from build123d import *

# Parameters (mm, degrees)
SKETCH1_R           = 1.397
SKETCH1_R_2         = 1.651
SKETCH1_R_3         = 1.016
SKETCH1_W           = 58.544107304
SKETCH1_H           = 8.89
SKETCH1_W_2         = 6.35
SKETCH1_H_2         = 3.175
BOSS_EXTRUDE1_DEPTH = 3.175


with BuildPart() as part:
    # Sketch1 → Boss-Extrude1 (new body)
    with BuildSketch(Plane(origin=(0, 0, 0), x_dir=(1, 0, 0), z_dir=(0, 1, 0))):
        with BuildLine():
            Line((38.407265908, 13.335), (41.582265908, 13.335))
            Line((41.582265908, 13.335), (50.342102347, 13.335))
            ThreePointArc((50.342102347, 13.335), (57.058059725, 24.74076345), (67.270928268, 33.160552015))
            ThreePointArc((67.270928268, 33.160552015), (-10.756431789, 74.224653419), (-73.916912814, 12.7))
            Line((-73.916912814, 12.7), (-73.916912814, -12.7))
            ThreePointArc((-73.916912814, -12.7), (-10.756431789, -74.224653419), (67.270928268, -33.160552015))
            ThreePointArc((67.270928268, -33.160552015), (60.584216496, -28.355013333), (55.086193863, -22.225))
            ThreePointArc((55.086193863, -22.225), (52.41895011, -17.937530518), (50.342102347, -13.335))
            Line((50.342102347, -13.335), (46.281265908, -13.335))
            Line((46.281265908, -13.335), (41.582265908, -13.335))
            Line((41.582265908, -13.335), (41.582265908, -22.86))
            Line((41.582265908, -22.86), (38.407265908, -22.86))
            Line((38.407265908, -22.86), (38.407265908, -13.335))
            Line((38.407265908, -13.335), (-2.486734092, -13.335))
            Line((-2.486734092, -13.335), (-2.486734092, -6.604))
            Line((-2.486734092, -6.604), (-38.046734092, -6.604))
            Line((-38.046734092, -6.604), (-38.046734092, 6.604))
            Line((-38.046734092, 6.604), (-2.486734092, 6.604))
            Line((-2.486734092, 6.604), (-2.486734092, 13.335))
            Line((-2.486734092, 13.335), (38.407265908, 13.335))
        make_face()
        with Locations(Location((-62.486912814, 6.731, 0), (0, 0, 270))):
            Circle(SKETCH1_R, mode=Mode.SUBTRACT)
        with Locations(Location((-62.486912814, -6.731, 0), (0, 0, 270))):
            Circle(SKETCH1_R, mode=Mode.SUBTRACT)
        with Locations(Location((-39.626912814, -48.698461806, 0), (0, 0, 270))):
            Circle(SKETCH1_R_2, mode=Mode.SUBTRACT)
        with Locations(Location((39.626912814, -48.698461806, 0), (0, 0, 270))):
            Circle(SKETCH1_R_2, mode=Mode.SUBTRACT)
        with Locations(Location((39.626912814, 48.698461806, 0), (0, 0, 90))):
            Circle(SKETCH1_R_2, mode=Mode.SUBTRACT)
        with Locations(Location((0, -24.638, 0), (0, 0, 270))):
            Circle(SKETCH1_R_2, mode=Mode.SUBTRACT)
        with Locations(Location((-39.626912814, 48.698461806, 0), (0, 0, 90))):
            Circle(SKETCH1_R_2, mode=Mode.SUBTRACT)
        with Locations(Location((0, 24.638, 0), (0, 0, 90))):
            Circle(SKETCH1_R_2, mode=Mode.SUBTRACT)
        with Locations(Location((29.272053652, -37.649461806, 0), (0, 0, 270))):
            Circle(SKETCH1_R, mode=Mode.SUBTRACT)
        with Locations(Location((-58.676912814, 34.29, 0), (0, 0, 270))):
            Circle(SKETCH1_R_2, mode=Mode.SUBTRACT)
        with Locations(Location((62.141053559, -35.830642926, 0), (0, 0, 270))):
            Circle(SKETCH1_R_3, mode=Mode.SUBTRACT)
        with Locations(Location((56.570777105, -32.679132142, 0), (0, 0, 270))):
            Circle(SKETCH1_R_3, mode=Mode.SUBTRACT)
        with Locations(Location((-58.676912814, -34.29, 0), (0, 0, 270))):
            Circle(SKETCH1_R_2, mode=Mode.SUBTRACT)
        with Locations(Location((29.272053652, -24.187461806, 0), (0, 0, 270))):
            Circle(SKETCH1_R, mode=Mode.SUBTRACT)
        with Locations(Location((29.272053652, 37.649461806, 0), (0, 0, 90))):
            Circle(SKETCH1_R, mode=Mode.SUBTRACT)
        with Locations(Location((29.272053652, 24.187461806, 0), (0, 0, 90))):
            Circle(SKETCH1_R, mode=Mode.SUBTRACT)
        with Locations(Location((62.141053559, 35.830642926, 0), (0, 0, 270))):
            Circle(SKETCH1_R_3, mode=Mode.SUBTRACT)
        with Locations(Location((56.570777105, 32.679132142, 0), (0, 0, 270))):
            Circle(SKETCH1_R_3, mode=Mode.SUBTRACT)
        with Locations(Location((22.278265908, 19.05, 0), (0, 0, 270))):
            Circle(SKETCH1_R_2, mode=Mode.SUBTRACT)
        with Locations(Location((22.278265908, -19.05, 0), (0, 0, 270))):
            Circle(SKETCH1_R_2, mode=Mode.SUBTRACT)
        with Locations(Location((-22.171734092, -19.05, 0), (0, 0, 270))):
            Circle(SKETCH1_R_2, mode=Mode.SUBTRACT)
        with Locations(Location((-22.171734092, 19.05, 0), (0, 0, 270))):
            Circle(SKETCH1_R_2, mode=Mode.SUBTRACT)
        with Locations((0, -61.144461806)):
            Rectangle(SKETCH1_W, SKETCH1_H, mode=Mode.SUBTRACT)
        with Locations((0, 61.144461806)):
            Rectangle(SKETCH1_W, SKETCH1_H, mode=Mode.SUBTRACT)
        with Locations((55.791053559, -40.593142926)):
            Rectangle(SKETCH1_W_2, SKETCH1_H_2, mode=Mode.SUBTRACT)
        with Locations((55.791053559, 40.593142926)):
            Rectangle(SKETCH1_W_2, SKETCH1_H_2, mode=Mode.SUBTRACT)
        Polygon((32.44100721, -56.895314679), (35.719111901, -62.333745485), (38.438327304, -60.694693139), (35.160222613, -55.256262334), align=None, mode=Mode.SUBTRACT)
        Polygon((-32.44100721, -56.895314679), (-35.160222613, -55.256262334), (-38.438327304, -60.694693139), (-35.719111901, -62.333745485), align=None, mode=Mode.SUBTRACT)
        Polygon((-35.160222613, 55.256262334), (-38.438327304, 60.694693139), (-35.719111901, 62.333745485), (-32.44100721, 56.895314679), align=None, mode=Mode.SUBTRACT)
        Polygon((35.160222613, 55.256262334), (38.438327304, 60.694693139), (35.719111901, 62.333745485), (32.44100721, 56.895314679), align=None, mode=Mode.SUBTRACT)
        with Locations((-67.566912814, 0)):
            Rectangle(SKETCH1_W_2, SKETCH1_H_2, mode=Mode.SUBTRACT)
    extrude(amount=BOSS_EXTRUDE1_DEPTH)


solid = part.part
Source: CAD feature listing. Evaluate the final solid. Frame: model axes, mm. A direction names the side the tool comes from. Coordinates: 2 decimals unless noted, no trailing zeros. Loops run counter-clockwise (first coordinate to the right, second up) from the corner with the lowest first, then second, coordinate; pieces in that order, holes last. Notation, with made-up numbers: (46.5, 57.25) - (70.5, 57.25) arc R20 ccw to (70.5, 90.25) - close; hole circle Ø9 at (32.5, 36.25). An arc over 180 degrees is marked (long way). Return JSON: item names as keys, results as strings.
Q1. Contact query for flat-ended pins moving along their axis: P1, Ø1.6, axis at y = 1, z = 2.5, coming from the +X side; P2, Ø1.6, axis at x = -68.5, y = 1.5, coming from the -Z side; P3, Ø1.6, axis at x = 55.5, y = 1, coming from the -Z side. Output: stop coordinate, or through.
Results:
{"P1": "x = -38.05", "P2": "z = -32.28", "P3": "z = -51.31"}
Q2. Section C-C, the plane y = 0.85. Give the number of separate pieces and of enclosed holes in the cut face, plus the area to 3 significant figures.
Results:
{"separate pieces": "1", "enclosed holes": "31", "area": "13,200 mm2"}
Q3. Section B-B, the plane z = 19.05. Return loops of the section in (x, y) (3 decimals).
Results:
{"outline": "(-72.54, 0) - (-23.823, 0) - (-23.823, 3.175) - (-72.54, 3.175) - close; (-20.521, 0) - (20.627, 0) - (20.627, 3.175) - (-20.521, 3.175) - close; (23.929, 0) - (38.407, 0) - (38.407, 3.175) - (23.929, 3.175) - close; (41.582, 0) - (53.037, 0) - (53.037, 3.175) - (41.582, 3.175) - close"}
Q4. Mould query, pull axis X, two halves, no side actions, for faces 1 (the cylindrical face through (-12.061, 1.565, 74.024)), 2 (the flat face through (58.966, 2, -41)), 3 (the flat face through (-2.487, 2, -10)). Classes: released by +X, released by -X, zero draft, split by the parting line, or undercut.
Results:
{"face 1": "split by the parting line", "face 2": "undercut", "face 3": "released by +X"}
Q5. Section A-A, the plane x = 0. Return loops of the section in (y, z) (3 decimals), plus the area to 3 significant figures.
Results:
{"outline": "(0, -75) - (3.175, -75) - (3.175, -65.589) - (0, -65.589) - close; (0, -56.699) - (3.175, -56.699) - (3.175, -26.289) - (0, -26.289) - close; (0, -22.987) - (3.175, -22.987) - (3.175, -13.335) - (0, -13.335) - close; (0, 13.335) - (3.175, 13.335) - (3.175, 22.987) - (0, 22.987) - close; (0, 26.289) - (3.175, 26.289) - (3.175, 56.699) - (0, 56.699) - close; (0, 65.589) - (3.175, 65.589) - (3.175, 75) - (0, 75) - close", "area": "314 mm2"}
Q6. Material intervals for line 1 along Z through (x, y) = (2, 2.3) (3 decimals); line 2 along X through (y, z) = (0.8, 7); line 3 along X through (y, z) = (2.9, -62), sorted ascending.
Results:
{"line 1": "-74.973 to -65.589, -56.699 to -13.335, 13.335 to 56.699, 65.589 to 74.973", "line 2": "-73.92 to -63.86, -61.12 to -2.49", "line 3": "-42.2 to -36.27, -35.52 to -29.27, 29.27 to 35.52, 36.27 to 42.2"}
Q7. Access query for faces 4 (the flat face through (-4, 3.175, 16)), 5 (the flat face through (-21, 2, -6.604)), 6 (the flat face through (29.272, 2, 61)). Directions: +Z, -Z, +X, -X, +Y, -Y. A direction counts if a zero-diameter tool reaches every point of the face in a straight line with its end or side. Return the directions, or none.
Results:
{"face 4": "+Z, -Z, +X, -X, +Y", "face 5": "+X, +Y, -Y", "face 6": "+Y, -Y"}
Q8. Section D-D, the plane z = -45. Return loops of the section in (x, y) (3 decimals), plus the area to 3 significant figures.
Results:
{"outline": "(-60, 0) - (60, 0) - (60, 3.175) - (-60, 3.175) - close", "area": "381 mm2"}
